Autodesk Inventor part; units mm, degrees
ref_plane "YZ Plane" through (0, 0, 0) normal (1, 0, 0) x (0, 1, 0)
ref_plane "XZ Plane" through (0, 0, 0) normal (0, 1, 0) x (-1, 0, 0)
ref_plane "XY Plane" through (0, 0, 0) normal (0, 0, 1) x (1, 0, 0)
sketch "Эскиз1" plane through (0, 0, 0) normal (0, 0, 1) x (1, 0, 0)
  circle A0 centre (-2.1207, -4.0482) radius 1.65
  circle A1 centre (2.1207, -5.1509) radius 1.65
  line L0 (-5.0242, 4.325) -> (-5.0242, -8.5)
  line L1 (5.0242, -8.5) -> (5.0242, 7.5)
  line L2 (5.0242, 7.5) -> (-1.8492, 7.5)
  circle A2 centre (-2.0244, 2.1263) radius 1.5
  arc A3 (-1.8492, 7.5) -> (-5.0242, 4.325) centre (-1.8492, 4.325) ccw
  line L3 (-5.0242, -8.5) -> (5.0242, -8.5)
  dimension "d0" = 3.175
  dimension "d1" = 3.3
  dimension "d2" = 3
  dimension "d3" = 3.3
extrude "Выдавливание1" add sketch "Эскиз1" along normal blind 5
properties part number "gates_top_holder"
Read the model definition and answer for the solid it produces. Units are mm, in the model's axes. Round coordinates to 2 decimals unless told otherwise and drop trailing zeros. Write each loop counter-clockwise with the first axis right and the second up, starting at its lowest first coordinate (ties: lowest second). Pieces come first, ordered by that corner, then holes.
Q1. Find section A-A on y = -4.25. Determine the outline of the cut face in (x, z).
Values:
outline: (-5.02, 0) - (-3.76, 0) - (-3.76, 5) - (-5.02, 5) - close; (-0.48, 0) - (0.74, 0) - (0.74, 5) - (-0.48, 5) - close; (3.5, 0) - (5.02, 0) - (5.02, 5) - (3.5, 5) - close
Q2. Find section D-D on x = -2.5. Determine the outline of the cut face in (y, z).
Values:
outline: (-8.5, 0) - (-5.65, 0) - (-5.65, 5) - (-8.5, 5) - close; (-2.44, 0) - (0.7, 0) - (0.7, 5) - (-2.44, 5) - close; (3.55, 0) - (7.43, 0) - (7.43, 5) - (3.55, 5) - close
Q3. Find section C-C on y = -6. Determine the outline of the cut face in (x, z), and give its area (3 significant figures).
Values:
outline: (-5.02, 0) - (0.71, 0) - (0.71, 5) - (-5.02, 5) - close; (3.54, 0) - (5.02, 0) - (5.02, 5) - (3.54, 5) - close
area: 36.1 mm2
Q4. Straight lines are drawn through the part: line 1 (Y direction, x = 2, z = 2.55); line 2 (X direction, y = -4.25, z = 2.1); line 3 (Y direction, x = -1.75, z = 1.8). For each, find the intervals that lie inside material, in ascending order.
Values:
line 1: y = -8.5 to -6.8, -3.51 to 7.5
line 2: x = -5.02 to -3.76, -0.48 to 0.74, 3.5 to 5.02
line 3: y = -8.5 to -5.66, -2.44 to 0.65, 3.6 to 7.5
Q5. Find section B-B on z = 2.3. Determine the outline of the cut face in (x, y) (3 decimals), and give its area (3 significant figures).
Values:
outline: (-5.024, -8.5) - (5.024, -8.5) - (5.024, 7.5) - (-1.849, 7.5) arc R3.175 ccw to (-5.024, 4.325) - close; hole circle Ø3.3 at (-2.121, -4.048); hole circle Ø3 at (-2.024, 2.126); hole circle Ø3.3 at (2.121, -5.151)
area: 134 mm2
